Part model, mm, in its own coordinate system. Face numbers are marked on the shaded views. A direction names the side the tool comes from. Round coordinates to 2 decimals unless told otherwise and drop trailing zeros. Loops run counter-clockwise (first coordinate to the right, second up) from the corner with the lowest first, then second, coordinate; pieces in that order, holes last.
1) Band-saw the part on A-A, the plane z = 32.5. Write the cut outline in (x, y), then the cut area to 3 significant figures.
2) Band-saw the part on C-C, the plane y = -5. Write the cut outline in (x, z), then the cut area to 3 significant figures.
3) Band-saw the part on B-B, the plane x = 22. Write the cut outline in (y, z).
4) Drop flat-ended pins along their axis: P1, Ø6, axis at y = -16, z = 43, coming from the -X side; P2, Ø7.5, axis at x = 15, y = -13.5, coming from the +Z side; P3, Ø12.5, axis at y = -8.5, z = -17, coming from the +X side; P4, Ø9.5, axis at x = 33.12, z = 10.53, coming from the +Y side. Give the stop position or say it passes through.
5) 3-axis set-ups, long thin cutter, end or side, ignore diameter. For the marked faces 1, 2 and 3: which of +Z, -Z, +X, -X, +Y, -Y reach the whole face in a straight line?
6) Probe line 1 (X direction, y = -2.5, z = -11); line 2 (Z direction, x = 36, y = -4.75); line 3 (X direction, y = -4.5, z = 47.5). List the from-to ranges inside material, lowest first.
7) Mould opens along X. For the marked faces 4, 5, 6 and 7 say: +X half, -X half, draft (parallel to the pull), parting line (faces both ways), or undercut.
from build123d import *

# Parameters (mm, degrees)
F0_R     = 10.571471
F0_R_2   = 7.723691
F0_R_3   = 3.821059
F1_DEPTH = 25.4


with BuildPart() as f1:
    # F0 (on Front) → F1 (new body)
    with BuildSketch(Plane.XZ):
        Polygon((0, 0), (0, -25.4), (25.4, -25.4), (25.4, 0), (50.8, 0), (50.8, 25.4), (50.8, 50.8), (25.4, 50.8), (25.4, 25.4), (0, 25.4), align=None)
        with Locations((13.713269, -10.571471)):
            Circle(F0_R, mode=Mode.SUBTRACT)
        with Locations((33.123691, 10.526813)):
            Circle(F0_R_2, mode=Mode.SUBTRACT)
        with Locations((37.343346, 33.734929)):
            Circle(F0_R_3, mode=Mode.SUBTRACT)
    extrude(amount=F1_DEPTH)


solid = f1.part
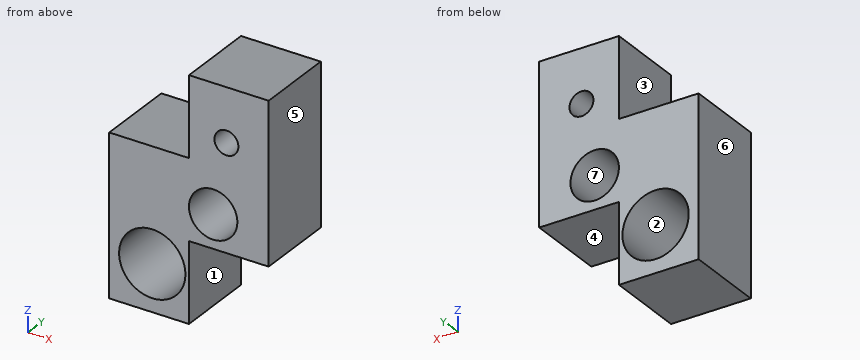
Reported:
1. outline: (25.4, -25.4) - (33.73, -25.4) - (33.73, 0) - (25.4, 0) - close; (40.96, -25.4) - (50.8, -25.4) - (50.8, 0) - (40.96, 0) - close
1. area: 461 mm2
2. outline: (0, -25.4) - (25.4, -25.4) - (25.4, 0) - (50.8, 0) - (50.8, 50.8) - (25.4, 50.8) - (25.4, 25.4) - (0, 25.4) - close; hole circle Ø21.14 at (13.71, -10.57); hole circle Ø15.45 at (33.12, 10.53); hole circle Ø7.64 at (37.34, 33.73)
2. area: 2,000 mm2
3. outline: (-25.4, -25.4) - (0, -25.4) - (0, -17.14) - (-25.4, -17.14) - close; (-25.4, -4.01) - (0, -4.01) - (0, 25.4) - (-25.4, 25.4) - close
4. P1: stops at x = 25.4
4. P2: stops at z = 25.4
4. P3: stops at x = 25.4
4. P4: passes through
5. face 1: -Z, +X, +Y, -Y
5. face 2: +Y, -Y
5. face 3: +Z, -X, +Y, -Y
6. line 1: x = 0 to 3.15, 24.28 to 25.4
6. line 2: z = 0 to 3.36, 17.69 to 30.16, 37.31 to 50.8
6. line 3: x = 25.4 to 50.8
7. face 4: draft
7. face 5: +X half
7. face 6: -X half
7. face 7: undercut
